from build123d import *

# Parameters (mm, degrees)
SKETCH1_R           = 3.1
BOSS_EXTRUDE1_DEPTH = 4.5


with BuildPart() as part:
    # Sketch1 → Boss-Extrude1 (new body)
    with BuildSketch(Plane(origin=(0, 0, 0), x_dir=(1, 0, 0), z_dir=(0, 1, 0))):
        with BuildLine():
            Line((10, 0), (25, 0))
            Line((25, 0), (28.5, 0))
            ThreePointArc((28.5, 0), (29.207106781, 0.292893219), (29.5, 1))
            Line((29.5, 1), (29.5, 9))
            ThreePointArc((29.5, 9), (29.207106781, 9.707106781), (28.5, 10))
            Line((28.5, 10), (25, 10))
            Line((25, 10), (25, 15))
            Line((25, 15), (28.5, 15))
            ThreePointArc((28.5, 15), (29.207106781, 15.292893219), (29.5, 16))
            Line((29.5, 16), (29.5, 24))
            ThreePointArc((29.5, 24), (29.207106781, 24.707106781), (28.5, 25))
            Line((28.5, 25), (25, 25))
            Line((25, 25), (10, 25))
            ThreePointArc((10, 25), (2.928932188, 22.071067812), (0, 15))
            Line((0, 15), (0, 10))
            ThreePointArc((0, 10), (2.928932188, 2.928932188), (10, 0))
        make_face()
        with Locations(Location((10, 12.5, 0), (0, 0, 270))):
            Circle(SKETCH1_R, mode=Mode.SUBTRACT)
    extrude(amount=BOSS_EXTRUDE1_DEPTH)


solid = part.part
CAD build for the part. Positions are in the model's coordinates, mm. A direction names the side the tool comes from. Round coordinates to 2 decimals unless told otherwise and drop trailing zeros. Write each loop counter-clockwise with the first axis right and the second up, starting at its lowest first coordinate (ties: lowest second). Pieces come first, ordered by that corner, then holes. Notation, with made-up numbers: M -30.75,-13 L 5.25,-13 A6 ccw 5.25,-7 Z; hole C -18,79.5 d8. An arc over 180 degrees is marked long. Put each result on its own line as item: value. Start each with the question number.
1) 3-axis set-ups, long thin cutter, end or side, ignore diameter. For faces 4 (the flat face through (27, 2, -15)), 5 (the flat face through (29.5, 2, -5)): which of +Z, -Z, +X, -X, +Y, -Y reach the whole face in a straight line?
2) Pull direction X, two halves, no side cores. Call faces 1 (the cylindrical face through (10.1, 2.2, -15.6)), 2 (the flat face through (15, 4.5, -13)), 3 (the cylindrical face through (29.215, 2.218, -9.699)): pulls with the +X half, pulls with the -X half, needs draft (parallel to the pull), parting line crosses it, or undercut.
3) Drill centre lines: probe 1 along X at (y, z) = (1.5, -12.5); probe 2 along X at (y, z) = (3.3, -14); probe 3 along X at (y, z) = (3.85, -1.5). Where is each one in solid material? Low to high. Write a range as [from, to].
4) Saw through at D-D, the plane x = 4.5. Write the cut outline in (y, z).
5) Saw through at A-A, the plane z = -12.5. Write the cut outline in (x, y).
6) Pin check, flat tips, straight feed: pin 1 Ø1.3 at (y, z) = (2, -13.5) entering from +X; pin 2 Ø1.5 at (y, z) = (2, -16) entering from -X. Stop position of each tip, or through.
7) Saw through at B-B, the plane y = 1.6. Write the cut outline in (x, z), and give its area (3 significant figures).
8) Saw through at C-C, the plane x = 9.25. Write the cut outline in (y, z), and give its area (3 significant figures).
Resolved:
1. face 4: +X, +Y, -Y
1. face 5: +Z, -Z, +X, +Y, -Y
2. face 1: undercut
2. face 2: needs draft
2. face 3: pulls with the +X half
3. probe 1: [0, 6.9], [13.1, 25]
3. probe 2: [0, 7.29], [12.71, 25]
3. probe 3: [4.73, 29.5]
4. outline: M 0,-23.35 L 4.5,-23.35 L 4.5,-1.65 L 0,-1.65 Z
5. outline: M 0,0 L 6.9,0 L 6.9,4.5 L 0,4.5 Z; M 13.1,0 L 25,0 L 25,4.5 L 13.1,4.5 Z
6. pin 1: x = 25
6. pin 2: x = 0
7. outline: M 0,-15 A10 ccw 10,-25 L 28.5,-25 A1 ccw 29.5,-24 L 29.5,-16 A1 ccw 28.5,-15 L 25,-15 L 25,-10 L 28.5,-10 A1 ccw 29.5,-9 L 29.5,-1 A1 ccw 28.5,0 L 10,0 A10 ccw 0,-10 Z; hole C 10,-12.5 d6.2
7. area: 641 mm²
8. outline: M 0,-24.97 L 4.5,-24.97 L 4.5,-15.51 L 0,-15.51 Z; M 0,-9.49 L 4.5,-9.49 L 4.5,-0.03 L 0,-0.03 Z
8. area: 85.2 mm²
